Input: part model. Units: mm. Frame: model coordinates. A direction names the side the tool comes from. Give positions to 0.01 mm unless a question says otherwise; leave off trailing zeros. Order: outer loops, then holes, each group sorted by start corner. A loop starts at its lowest first (then second) coordinate and runs counter-clockwise, first axis right, second up. Notation, with made-up numbers: M -1,36 L 21,36 A30 cw 21,73 Z; hole C 24,9.5 d4. An arc over 180 degrees is marked long. Use a Markdown table: item, result.
from build123d import *

# Parameters (mm, degrees)
BOSS_EXTRU_1_DEPTH      = 5
ESQUISSE3_W             = 10
ESQUISSE3_H             = 3
ENL_V_MAT_EXTRU_1_DEPTH = 231.967242256
ENL_V_MAT_EXTRU_2_DEPTH = 231.967242256
ESQUISSE2_W             = 203.424903091
ESQUISSE2_H             = 131.549645995
ENL_V_MAT_EXTRU_3_DEPTH = 231.967242256
CONG_1_R                = 2.5
ESQUISSE5_W             = 4
ESQUISSE5_H             = 10
ENL_V_MAT_EXTRU_4_DEPTH = 206.267190359


with BuildPart() as part:
    # Esquisse1 → Boss.-Extru.1 (new body)
    with BuildSketch(Plane.XY):
        with BuildLine():
            Line((0, 0), (0, -25))
            Line((0, -25), (37.5, -25))
            Line((37.5, -25), (37.5, -95.5))
            Line((37.5, -95.5), (32.5, -95.5))
            Line((32.5, -95.5), (36.487358688, -115.098494092))
            Line((36.487358688, -115.098494092), (88.487358688, -115.098494092))
            Line((88.487358688, -115.098494092), (159.198036807, -44.387815974))
            ThreePointArc((159.198036807, -44.387815974), (187.146342861, -3.044299659), (200.182925478, 45.126663235))
            Line((200.182925478, 45.126663235), (43.682925478, 43.998857528))
            ThreePointArc((43.682925478, 43.998857528), (12.775400091, 31.000392909), (0, 0))
        make_face()
    extrude(amount=BOSS_EXTRU_1_DEPTH)

    # Esquisse3 → Enlèv. mat.-Extru.1 (cut, through all)
    with BuildSketch(Plane.XY.offset(5)):
        with Locations((5, -23.5)):
            Rectangle(ESQUISSE3_W, ESQUISSE3_H)
    extrude(amount=-ENL_V_MAT_EXTRU_1_DEPTH, mode=Mode.SUBTRACT)

    # Esquisse4 → Enlèv. mat.-Extru.2 (cut, through all)
    with BuildSketch(Plane.XY.offset(5)):
        Polygon((88.487358688, -105.098494092), (78.487358688, -105.098494092), (78.487358688, -111.098494092), (68.487358688, -115.098494092), (78.487358688, -115.098494092), (88.487358688, -115.098494092), (98.487358688, -105.098494092), align=None)
    extrude(amount=-ENL_V_MAT_EXTRU_2_DEPTH, mode=Mode.SUBTRACT)

    # Esquisse2 → Enlèv. mat.-Extru.3 (cut, through all)
    with BuildSketch(Plane.XY.offset(5)):
        with Locations((101.712451546, -70.774822998)):
            Rectangle(ESQUISSE2_W, ESQUISSE2_H)
    extrude(amount=-ENL_V_MAT_EXTRU_3_DEPTH, mode=Mode.SUBTRACT)

    # Congé1
    cong_1_edges = [part.edges().sort_by_distance(p)[0] for p in [
        (93.117022594, -5, 0),
        (93.117022594, -5, 5),
    ]]
    fillet(cong_1_edges, radius=CONG_1_R - 0.0001)  # a hair under: the kernel refuses the full size

    # Esquisse5 → Enlèv. mat.-Extru.4 (cut, through all)
    with BuildSketch(Plane.XY.offset(5)):
        with Locations((57, 32.5)):
            Rectangle(ESQUISSE5_W, ESQUISSE5_H)
    extrude(amount=-ENL_V_MAT_EXTRU_4_DEPTH, mode=Mode.SUBTRACT)


solid = part.part
1) Reachability of faces 4 (the face through (99, 22, 5)), 5 (the face through (57, 37.5, 3)) from +Z, -Z, +X, -X, +Y, -Y: full face, straight path, thin tool, end or side. Return the list, or none.
Response values:
| item | result |
|---|---|
| face 4 | +Z, +X, -X, +Y, -Y |
| face 5 | +Z, -Z |
2) Cut plane A-A on y = 32.5. Return loops of the section in (x, z), and give its area (3 significant figures).
Response values:
| item | result |
|---|---|
| outline | M 14.34,0 L 55,0 L 55,5 L 14.34,5 Z; M 59,0 L 198.39,0 L 198.39,5 L 59,5 Z |
| area | 900 mm² |
3) Material intervals for line 1 (X direction, y = 34, z = 4.85); line 2 (X direction, y = 36, z = 1.9); line 3 (Y direction, x = 57, z = 3.6), sorted ascending. Write a range as from..to.
Response values:
| item | result |
|---|---|
| line 1 | x = 16.07..55, 59..198.66 |
| line 2 | x = 18.7..55, 59..198.99 |
| line 3 | y = -4.75..27.5, 37.5..44.09 |
4) Cut plane B-B on z = 1. Return loops of the section in (x, y), and give its area (3 significant figures).
Response values:
| item | result |
|---|---|
| outline | M 0,-4.5 L 186.47,-4.5 A151.85 ccw 200.18,45.13 L 43.68,44 A44 ccw 0,0 Z; hole M 55,27.5 L 59,27.5 L 59,37.5 L 55,37.5 Z |
| area | 9,080 mm² |
5) First-contact query: pin 1 Ø1.2 at (x, z) = (57.5, 2.5) entering from +Y; pin 2 Ø2 at (y, z) = (16, 3) entering from -X. Flat tips, straight axial feed; report the tip coordinate or a pass-through.
Response values:
| item | result |
|---|---|
| pin 1 | stops at y = 44.1 |
| pin 2 | stops at x = 2.64 |
6) Mould query, pull axis Y, two halves, no side actions, for faces 1 (the face through (55, 32, 3)), 2 (the face through (13.117, 31.34, 2.465)), 3 (the face through (0, -2, 2)). Classes: released by +Y, released by -Y, zero draft, split by the parting line, or undercut.
Response values:
| item | result |
|---|---|
| face 1 | undercut |
| face 2 | released by +Y |
| face 3 | zero draft |
7) Cut plane D-D on y = 13. Return loops of the section in (x, z), and give its area (3 significant figures).
Response values:
| item | result |
|---|---|
| outline | M 1.96,0 L 193.42,0 L 193.42,5 L 1.96,5 Z |
| area | 957 mm² |
